The listing builds one solid part. Answer for the finished solid, in the listing's coordinates (mm). Coordinates: 2 decimals unless noted, no trailing zeros. Order: outer loops, then holes, each group sorted by start corner. A loop starts at its lowest first (then second) coordinate and runs counter-clockwise, first axis right, second up. Notation, with made-up numbers: (84, -7) -> (122, -7) arc R17 ccw to (122, -3) -> close; hole circle Ø3 at (65.25, 68.25). An arc over 180 degrees is marked (long way). Write each question's results on one line, items separated by ' | '. Start each with the question number.
(1) The part is cut by section D-D, the plane x = 5.5. Give the vertices of the cut face in (y, z).
(2) The part is cut by section C-C, the plane y = 2.5. Give the vertices of the cut face in (x, z).
(3) The part is cut by section A-A, the plane y = -7. Give the vertices of the cut face in (x, z), then the cut area to 3 significant figures.
(4) Given pin 1 (3.5 mm diameter, centred on x = 0, z = 5, fed in from -Y); pin 2 (8.5 mm diameter, centred on x = 0, y = 4.5, fed in from +Z); pin 3 (5 mm diameter, centred on x = -4, y = -2.5, fed in from -Z), each flat-ended and moving along its own axis, determine where each tip first touches the part or whether it passes through.
(5) Straight lines are drawn through the part: L1, parallel to Z at x = 0, y = -5; L2, parallel to X at y = -8.75, z = 5; L3, parallel to Y at x = 2, z = 8.75. For each, find the intervals that lie inside material, in ascending order.
(6) The part is cut by section B-B, the plane x = -3.5. Give the vertices of the cut face in (y, z).
(7) Determine the mould class of faces 1 (the face through (0.273, -7.241, 7.082)), 2 (the face through (0, -2, 10)), 3 (the face through (8, -4, 5)) for opening direction X: +X half, -X half, draft (parallel to the pull), parting line (faces both ways), or undercut.
```python
from build123d import *

# Parameters (mm, degrees)
F0_R     = 5.25
F1_DEPTH = 10
F3_D     = 4.2
F3_DEPTH = 8.4
F3_TIP   = 1.2618073


with BuildPart() as f1:
    # F0 (on Top) → F1 (new body)
    with BuildSketch(Plane.XY):
        with BuildLine():
            Line((-8, -11.5), (8, -11.5))
            Line((8, -11.5), (8, 3.5))
            ThreePointArc((8, 3.5), (5.6568542495, 9.1568542495), (0, 11.5))
            ThreePointArc((0, 11.5), (-5.6568542495, 9.1568542495), (-8, 3.5))
            Line((-8, 3.5), (-8, -11.5))
        make_face()
        with Locations((0, 4.5)):
            Circle(F0_R, mode=Mode.SUBTRACT)
    extrude(amount=F1_DEPTH)

    # F3
    with Locations(Plane.XZ.offset(11.5)):
        with Locations((0, 5)):
            Hole(F3_D / 2, depth=F3_DEPTH)
            with Locations((0, 0, -(F3_DEPTH + F3_TIP / 2))):  # 118° drill point
                Cone(0, F3_D / 2, F3_TIP, mode=Mode.SUBTRACT)


solid = f1.part
```
Established:
1) outline: (-11.5, 0) -> (9.31, 0) -> (9.31, 10) -> (-11.5, 10) -> close
2) outline: (-8, 0) -> (-4.85, 0) -> (-4.85, 10) -> (-8, 10) -> close; (4.85, 0) -> (8, 0) -> (8, 10) -> (4.85, 10) -> close
3) outline: (-8, 0) -> (8, 0) -> (8, 10) -> (-8, 10) -> close; hole circle Ø4.2 at (0, 5) | area: 146 mm^2
4) pin 1: stops at y = -2.89 | pin 2: passes through | pin 3: stops at z = 0
5) L1: z = 0 to 2.9, 7.1 to 10 | L2: x = -8 to -2.1, 2.1 to 8 | L3: y = -11.5 to -0.35, 9.35 to 11.25
6) outline: (-11.5, 0) -> (0.59, 0) -> (0.59, 10) -> (-11.5, 10) -> close; (8.41, 0) -> (10.69, 0) -> (10.69, 10) -> (8.41, 10) -> close
7) face 1: undercut | face 2: draft | face 3: +X half
